The listing builds one solid part. Answer for the finished solid, in the listing's coordinates (mm). A direction names the side the tool comes from. Coordinates: 2 decimals unless noted, no trailing zeros. Order: outer loops, then holes, each group sorted by start corner. A loop starts at its lowest first (then second) coordinate and runs counter-clockwise, first axis right, second up. Notation, with made-up numbers: (33, 39) -> (80, 39) arc R21 cw to (80, 49) -> close; hole circle Ø3 at (1.5, -24.75). An arc over 180 degrees is marked (long way). Answer in a Markdown table with one row per item. Add a question column.
```python
from build123d import *

# Parameters (mm, degrees)
BACKER_MAIN_R              = 15.24
BOSS_EXTRUDE1_DEPTH        = 6.35
SUBSTRATE_BACK_CLEARANCE_R = 11.938
CUT_EXTRUDE1_DEPTH         = 1.27
SUBSTRATE_CSINK_R          = 12.827
CUT_EXTRUDE2_DEPTH         = 1.016
SPRING_HOLE_R              = 4.7625
CUT_EXTRUDE3_DEPTH         = 3.175


with BuildPart() as part:
    # Backer Main → Boss-Extrude1 (new body)
    with BuildSketch(Plane.XY):
        Circle(BACKER_MAIN_R)
    extrude(amount=-BOSS_EXTRUDE1_DEPTH)

    # Substrate Back Clearance → Cut-Extrude1 (cut)
    with BuildSketch(Plane.XY):
        Circle(SUBSTRATE_BACK_CLEARANCE_R)
    extrude(amount=-CUT_EXTRUDE1_DEPTH, mode=Mode.SUBTRACT)

    # Substrate CSink → Cut-Extrude2 (cut)
    with BuildSketch(Plane.XY):
        Circle(SUBSTRATE_CSINK_R)
    extrude(amount=-CUT_EXTRUDE2_DEPTH, mode=Mode.SUBTRACT)

    # Spring Hole → Cut-Extrude3 (cut)
    with BuildSketch(Plane(origin=(0, 0, -6.35), x_dir=(-1, 0, 0), z_dir=(0, 0, -1))):
        Circle(SPRING_HOLE_R)
    extrude(amount=-CUT_EXTRUDE3_DEPTH, mode=Mode.SUBTRACT)


solid = part.part
```
Q1. Straight lines are drawn through the part: line 1 (Y direction, x = 0, z = -1.15); line 2 (Y direction, x = 0, z = -4); line 3 (Z direction, x = -5, y = 9.5). For each, find the intervals that lie inside material, in ascending order.
Q2. A cutting plane is placed at C-C (z = -2.5). Determine the outline of the cut face in (x, y).
Q3. A cutting plane is placed at D-D (y = 9). Determine the outline of the cut face in (x, z).
Q4. Determine the mould class of faces 4 (the face through (-7, -11, 0)), 5 (the face through (-3.3, -14.88, -3.13)), 6 (the face through (12.235, 3.853, -0.501)) for opening direction Y: +Y half, -Y half, draft (parallel to the pull), parting line (faces both ways), or undercut.
Q5. For faces 1 (the face through (3.78, -2.9, -4.78)), 2 (the face through (0, 0, -1.27)), 3 (the face through (3, 4, -6.35)), determine the directions among +Z, -Z, +X, -X, +Y, -Y from which every point of the face is accessible in a straight line to the end or side of a thin tool.
Q6. Given pin 1 (1 mm diameter, centred on y = 11.5, z = -3.5, fed in from -X); pin 2 (1.5 mm diameter, centred on y = -8, z = -3.5, fed in from -X); pin 3 (3 mm diameter, centred on x = -1.5, y = -1.5, fed in from -Z) (3 decimals), each flat-ended and moving along its own axis, determine where each tip first touches the part or whether it passes through.
Returned:
| question | item | result |
|---|---|---|
| 1 | line 1 | y = -15.24 to -11.94, 11.94 to 15.24 |
| 1 | line 2 | y = -15.24 to -4.76, 4.76 to 15.24 |
| 1 | line 3 | z = -6.35 to -1.27 |
| 2 | outline | circle Ø30.48 at (0, 0) |
| 3 | outline | (-12.3, -6.35) -> (12.3, -6.35) -> (12.3, 0) -> (9.14, 0) -> (9.14, -1.02) -> (7.84, -1.02) -> (7.84, -1.27) -> (-7.84, -1.27) -> (-7.84, -1.02) -> (-9.14, -1.02) -> (-9.14, 0) -> (-12.3, 0) -> close |
| 4 | face 4 | draft |
| 4 | face 5 | parting line |
| 4 | face 6 | undercut |
| 5 | face 1 | -Z |
| 5 | face 2 | +Z |
| 5 | face 3 | -Z, +X, -X, +Y, -Y |
| 6 | pin 1 | stops at x = -10.55 |
| 6 | pin 2 | stops at x = -13.41 |
| 6 | pin 3 | stops at z = -3.175 |
